```python
from build123d import *

# Parameters (mm, degrees)
EXTRUDE_THIN1_DEPTH     = 25.4
F_3_8_CLEARANCE_HOLE1_D = 10.0838
SKETCH4_W               = 38.1
SKETCH4_H               = 12.7
CUT_EXTRUDE1_DEPTH      = 3.54


with BuildPart() as part:
    # Sketch1 → Extrude-Thin1 (new body, symmetric)
    with BuildSketch(Plane.XY):
        with BuildLine():
            Line((-26.67, -53.34), (-26.67, -5.08))
            ThreePointArc((-26.67, -5.08), (-25.182102448, -1.487897552), (-21.59, 0))
            Line((-21.59, 0), (21.59, 0))
            ThreePointArc((21.59, 0), (25.182102448, -1.487897552), (26.67, -5.08))
            Line((26.67, -5.08), (26.67, -53.34))
            Line((26.67, -53.34), (24.13, -53.34))
            Line((24.13, -53.34), (24.13, -5.08))
            ThreePointArc((24.13, -5.08), (23.386051224, -3.283948776), (21.59, -2.54))
            Line((21.59, -2.54), (-21.59, -2.54))
            ThreePointArc((-21.59, -2.54), (-23.386051224, -3.283948776), (-24.13, -5.08))
            Line((-24.13, -5.08), (-24.13, -53.34))
            Line((-24.13, -53.34), (-26.67, -53.34))
        make_face()
    extrude(amount=EXTRUDE_THIN1_DEPTH, both=True)

    # 3/8 Clearance Hole1 (through all)
    with Locations(Plane(origin=(26.67, 0, 0), x_dir=(0, 0, -1), z_dir=(1, 0, 0))):
        with Locations((0, -31.75)):
            Hole(F_3_8_CLEARANCE_HOLE1_D / 2)

    # Sketch4 → Cut-Extrude1 (cut, through all)
    with BuildSketch(Plane.XZ.offset(2.54)):
        with Locations((0, 19.05)):
            Rectangle(SKETCH4_W, SKETCH4_H)
    extrude(amount=-CUT_EXTRUDE1_DEPTH, mode=Mode.SUBTRACT)


solid = part.part
```
Could you check a few things on this model? Use its own coordinates, in mm. A direction names the side the tool comes from. Coordinates: 2 decimals unless noted, no trailing zeros. Write each loop counter-clockwise with the first axis right and the second up, starting at its lowest first coordinate (ties: lowest second). Pieces come first, ordered by that corner, then holes. Notation, with made-up numbers: (-4.5, 46) - (30.5, 46) arc R20 cw to (30.5, 58) - close; hole circle Ø8 at (-26, 69). An arc over 180 degrees is marked (long way). Use a Markdown table: item, result.
Q1. Imagine slicing it at D-D (z = -1.5). List the corners of the cut face in (x, y) for me.
Geometry check:
| item | result |
|---|---|
| outline | (-26.67, -53.34) - (-24.13, -53.34) - (-24.13, -36.56) - (-26.67, -36.56) - close; (-26.67, -26.94) - (-24.13, -26.94) - (-24.13, -5.08) arc R2.54 cw to (-21.59, -2.54) - (21.59, -2.54) arc R2.54 cw to (24.13, -5.08) - (24.13, -26.94) - (26.67, -26.94) - (26.67, -5.08) arc R5.08 ccw to (21.59, 0) - (-21.59, 0) arc R5.08 ccw to (-26.67, -5.08) - close; (24.13, -53.34) - (26.67, -53.34) - (26.67, -36.56) - (24.13, -36.56) - close |
Q2. I'm going to push flat-ended pins straight in: pin 1 Ø2 at (y, z) = (-1.5, 20) entering from +X; pin 2 Ø11.5 at (y, z) = (-31.75, 0) entering from +X; pin 3 Ø1 at (x, z) = (-16.5, -19.5) entering from -Y; pin 4 Ø3 at (y, z) = (-1, 16) entering from -X. Where does each tip first touch, or does it pass through?
Geometry check:
| item | result |
|---|---|
| pin 1 | stops at x = 25.97 |
| pin 2 | stops at x = 26.67 |
| pin 3 | stops at y = -2.54 |
| pin 4 | stops at x = -25.97 |
Q3. Imagine slicing it at A-A (y = -31.75). List the corners of the cut face in (x, z) for me.
Geometry check:
| item | result |
|---|---|
| outline | (-26.67, -25.4) - (-24.13, -25.4) - (-24.13, -5.04) - (-26.67, -5.04) - close; (-26.67, 5.04) - (-24.13, 5.04) - (-24.13, 25.4) - (-26.67, 25.4) - close; (24.13, -25.4) - (26.67, -25.4) - (26.67, -5.04) - (24.13, -5.04) - close; (24.13, 5.04) - (26.67, 5.04) - (26.67, 25.4) - (24.13, 25.4) - close |
Q4. Imagine slicing it at B-B (y = -6.5). List the corners of the cut face in (x, z) for me, and give its area (3 significant figures).
Geometry check:
| item | result |
|---|---|
| outline | (-26.67, -25.4) - (-24.13, -25.4) - (-24.13, 25.4) - (-26.67, 25.4) - close; (24.13, -25.4) - (26.67, -25.4) - (26.67, 25.4) - (24.13, 25.4) - close |
| area | 258 mm2 |
Q5. Imagine slicing it at C-C (z = 13.5). List the corners of the cut face in (x, y) for me.
Geometry check:
| item | result |
|---|---|
| outline | (-26.67, -53.34) - (-24.13, -53.34) - (-24.13, -5.08) arc R2.54 cw to (-21.59, -2.54) - (-19.05, -2.54) - (-19.05, 0) - (-21.59, 0) arc R5.08 ccw to (-26.67, -5.08) - close; (19.05, -2.54) - (21.59, -2.54) arc R2.54 cw to (24.13, -5.08) - (24.13, -53.34) - (26.67, -53.34) - (26.67, -5.08) arc R5.08 ccw to (21.59, 0) - (19.05, 0) - close |
Q6. Thinking about a two-plate mould opening in X: for faces 1 (the cylindrical face through (-23.4, -3.3, 0.4)), 2 (the cylindrical face through (25.142, -1.449, 0.356)), 3 (the flat face through (-26.67, -24, 0)), 4 (the flat face through (26, -27, 25.4)), which applies, +X half, -X half, draft (parallel to the pull), parting line (faces both ways), or undercut?
Geometry check:
| item | result |
|---|---|
| face 1 | undercut |
| face 2 | +X half |
| face 3 | -X half |
| face 4 | draft |
Q7. Which directions (+Z, -Z, +X, -X, +Y, -Y) give clear straight access to the entire face, cutting with the end or side of a thin tool? Please do faces 5 (the flat face through (-24.13, -24, 0)), 6 (the flat face through (0, 0, -5)), 7 (the flat face through (-19.05, -1, 19)).
Geometry check:
| item | result |
|---|---|
| face 5 | +Z, -Z, -Y |
| face 6 | +Z, -Z, +X, -X, +Y |
| face 7 | +Z, +Y, -Y |
Q8. Please list where these lines run through material, in increasing order: L1, parallel to X at y = -24, z = 12; L2, parallel to Y at x = 0, z = -19.5; L3, parallel to X at y = -2.5, z = -16.
Geometry check:
| item | result |
|---|---|
| L1 | x = -26.67 to -24.13, 24.13 to 26.67 |
| L2 | y = -2.54 to 0 |
| L3 | x = -25.97 to 25.97 |
